from build123d import *

# Parameters (mm, degrees)
SKETCH1_W          = 51.5
SKETCH1_H          = 48.5
BASE_DEPTH         = 1.5
SKETCH1_6_W        = 51.5
SKETCH1_6_H        = 48.5
WALLS_DEPTH        = 17
SCREWS_START       = 11
SKETCH1_7_R        = 1
SKETCH1_7_W        = 1.5
SKETCH1_7_H        = 3
SKETCH1_7_H_2      = 4
SCREWS_DEPTH       = 1.5
TOP_START          = 15.5
SKETCH1_8_W        = 39.5
SKETCH1_8_H        = 3
SKETCH1_8_H_2      = 4
TOP_DEPTH          = 1.5
FILLET1_R          = 5
FILLET3_R          = 4
SKETCH2_R          = 4
CUT_EXTRUDE1_DEPTH = 1.5


with BuildPart() as part:
    # Sketch1 → base (new body)
    with BuildSketch(Plane(origin=(0, 0, 0), x_dir=(1, 0, 0), z_dir=(0, 1, 0))):
        with Locations((24.25, 22.75)):
            Rectangle(SKETCH1_W, SKETCH1_H)
    extrude(amount=BASE_DEPTH)

    # Sketch1<6> → walls (add)
    with BuildSketch(Plane(origin=(0, 0, 0), x_dir=(1, 0, 0), z_dir=(0, 1, 0))):
        with Locations((24.25, 22.75)):
            Rectangle(SKETCH1_6_W, SKETCH1_6_H)
        Polygon((4.5, 0), (0, 0), (0, 4.5), (0, 6), (0, 39.5), (0, 41), (0, 45.5), (4.5, 45.5), (6, 45.5), (42.5, 45.5), (44, 45.5), (48.5, 45.5), (48.5, 41), (48.5, 39.5), (48.5, 6), (48.5, 4.5), (48.5, 0), (44, 0), (42.5, 0), (6, 0), align=None, mode=Mode.SUBTRACT)
    extrude(amount=WALLS_DEPTH)

    # Sketch1<7> → screws (add)
    # profile 1 of 12: a face of its own
    with BuildSketch(Plane(origin=(0, 0, 0), x_dir=(1, 0, 0), z_dir=(0, 1, 0)).offset(SCREWS_START)):
        Polygon((44, 3), (44, 0), (48.5, 0), (48.5, 4.5), (44, 4.5), align=None)
        with Locations(Location((46.25, 2.25, 0), (0, 0, 270))):
            Circle(SKETCH1_7_R, mode=Mode.SUBTRACT)
    # profile 2 of 12: a face of its own
    with BuildSketch(Plane(origin=(0, 0, 0), x_dir=(1, 0, 0), z_dir=(0, 1, 0)).offset(SCREWS_START)):
        Polygon((42.5, 6), (42.5, 3), (44, 3), (44, 4.5), (48.5, 4.5), (48.5, 6), align=None)
    # profile 3 of 12: a face of its own
    with BuildSketch(Plane(origin=(0, 0, 0), x_dir=(1, 0, 0), z_dir=(0, 1, 0)).offset(SCREWS_START)):
        with Locations((43.25, 1.5)):
            Rectangle(SKETCH1_7_W, SKETCH1_7_H)
    # profile 4 of 12: a face of its own
    with BuildSketch(Plane(origin=(0, 0, 0), x_dir=(1, 0, 0), z_dir=(0, 1, 0)).offset(SCREWS_START)):
        Polygon((44, 41.5), (42.5, 41.5), (42.5, 39.5), (48.5, 39.5), (48.5, 41), (44, 41), align=None)
    # profile 5 of 12: a face of its own
    with BuildSketch(Plane(origin=(0, 0, 0), x_dir=(1, 0, 0), z_dir=(0, 1, 0)).offset(SCREWS_START)):
        Polygon((44, 45.5), (44, 41.5), (44, 41), (48.5, 41), (48.5, 45.5), align=None)
        with Locations(Location((46.25, 43.25, 0), (0, 0, 270))):
            Circle(SKETCH1_7_R, mode=Mode.SUBTRACT)
    # profile 6 of 12: a face of its own
    with BuildSketch(Plane(origin=(0, 0, 0), x_dir=(1, 0, 0), z_dir=(0, 1, 0)).offset(SCREWS_START)):
        with Locations((43.25, 43.5)):
            Rectangle(SKETCH1_7_W, SKETCH1_7_H_2)
    # profile 7 of 12: a face of its own
    with BuildSketch(Plane(origin=(0, 0, 0), x_dir=(1, 0, 0), z_dir=(0, 1, 0)).offset(SCREWS_START)):
        Polygon((0, 41), (0, 39.5), (6, 39.5), (6, 41.5), (4.5, 41.5), (4.5, 41), align=None)
    # profile 8 of 12: a face of its own
    with BuildSketch(Plane(origin=(0, 0, 0), x_dir=(1, 0, 0), z_dir=(0, 1, 0)).offset(SCREWS_START)):
        Polygon((0, 45.5), (0, 41), (4.5, 41), (4.5, 41.5), (4.5, 45.5), align=None)
        with Locations(Location((2.25, 43.25, 0), (0, 0, 270))):
            Circle(SKETCH1_7_R, mode=Mode.SUBTRACT)
    # profile 9 of 12: a face of its own
    with BuildSketch(Plane(origin=(0, 0, 0), x_dir=(1, 0, 0), z_dir=(0, 1, 0)).offset(SCREWS_START)):
        with Locations((5.25, 43.5)):
            Rectangle(SKETCH1_7_W, SKETCH1_7_H_2)
    # profile 10 of 12: a face of its own
    with BuildSketch(Plane(origin=(0, 0, 0), x_dir=(1, 0, 0), z_dir=(0, 1, 0)).offset(SCREWS_START)):
        Polygon((0, 4.5), (0, 0), (4.5, 0), (4.5, 3), (4.5, 4.5), align=None)
        with Locations(Location((2.25, 2.25, 0), (0, 0, 270))):
            Circle(SKETCH1_7_R, mode=Mode.SUBTRACT)
    # profile 11 of 12: a face of its own
    with BuildSketch(Plane(origin=(0, 0, 0), x_dir=(1, 0, 0), z_dir=(0, 1, 0)).offset(SCREWS_START)):
        Polygon((0, 6), (0, 4.5), (4.5, 4.5), (4.5, 3), (6, 3), (6, 6), align=None)
    # profile 12 of 12: a face of its own
    with BuildSketch(Plane(origin=(0, 0, 0), x_dir=(1, 0, 0), z_dir=(0, 1, 0)).offset(SCREWS_START)):
        with Locations((5.25, 1.5)):
            Rectangle(SKETCH1_7_W, SKETCH1_7_H)
    extrude(amount=SCREWS_DEPTH)

    # Sketch1<8> → top (add)
    with BuildSketch(Plane(origin=(0, 0, 0), x_dir=(1, 0, 0), z_dir=(0, 1, 0)).offset(TOP_START)):
        with Locations((24.25, 1.5)):
            Rectangle(SKETCH1_8_W, SKETCH1_8_H)
        with Locations((24.25, 43.5)):
            Rectangle(SKETCH1_8_W, SKETCH1_8_H_2)
    extrude(amount=TOP_DEPTH)

    # Fillet1
    # the kernel refuses this fillet: 5 mm, written as the material it adds along each edge
    with BuildSketch(Plane(origin=(0, 11, 0), x_dir=(0, -1, 0), z_dir=(1, 0, 0))) as fillet1_piece_1_section:
        with BuildLine():
            CenterArc((FILLET1_R, FILLET1_R), FILLET1_R, 180, 90)
            Line((0, FILLET1_R), (0, 0))
            Line((0, 0), (FILLET1_R, 0))
        make_face()
    fillet1_piece_1 = extrude(amount=6, mode=Mode.PRIVATE)
    fillet1_piece_1 = fillet1_piece_1 - Plane(origin=(2.25, 9.80856061, -2.25), x_dir=(0, 0, 1), z_dir=(0, -1, 0)) * Cylinder(1, 33, mode=Mode.PRIVATE)
    add(fillet1_piece_1)
    with BuildSketch(Plane(origin=(0, 11, -6), x_dir=(0, -1, 0), z_dir=(0, 0, 1))) as fillet1_piece_2_section:
        with BuildLine():
            CenterArc((FILLET1_R, FILLET1_R), FILLET1_R, 180, 90)
            Line((0, FILLET1_R), (0, 0))
            Line((0, 0), (FILLET1_R, 0))
        make_face()
    fillet1_piece_2 = extrude(amount=6, mode=Mode.PRIVATE)
    fillet1_piece_2 = fillet1_piece_2 - Plane(origin=(2.25, 9.808553236, -2.25), x_dir=(0, 0, 1), z_dir=(0, -1, 0)) * Cylinder(1, 32, mode=Mode.PRIVATE)
    add(fillet1_piece_2)
    with BuildSketch(Plane(origin=(0, 11, -45.5), x_dir=(0, -1, 0), z_dir=(0, 0, 1))) as fillet1_piece_3_section:
        with BuildLine():
            CenterArc((FILLET1_R, FILLET1_R), FILLET1_R, 180, 90)
            Line((0, FILLET1_R), (0, 0))
            Line((0, 0), (FILLET1_R, 0))
        make_face()
    fillet1_piece_3 = extrude(amount=6, mode=Mode.PRIVATE)
    fillet1_piece_3 = fillet1_piece_3 - Plane(origin=(2.25, 9.808553112, -43.25), x_dir=(0, 0, 1), z_dir=(0, -1, 0)) * Cylinder(1, 32, mode=Mode.PRIVATE)
    add(fillet1_piece_3)
    with BuildSketch(Plane(origin=(0, 11, -45.5), x_dir=(0, -1, 0), z_dir=(1, 0, 0))) as fillet1_piece_4_section:
        with BuildLine():
            CenterArc((FILLET1_R, -FILLET1_R), FILLET1_R, 90, 90)
            Line((0, -FILLET1_R), (0, 0))
            Line((0, 0), (FILLET1_R, 0))
        make_face()
    fillet1_piece_4 = extrude(amount=6, mode=Mode.PRIVATE)
    fillet1_piece_4 = fillet1_piece_4 - Plane(origin=(2.25, 9.808558943, -43.25), x_dir=(0, 0, 1), z_dir=(0, -1, 0)) * Cylinder(1, 33, mode=Mode.PRIVATE)
    add(fillet1_piece_4)
    with BuildSketch(Plane(origin=(48.5, 11, -45.5), x_dir=(0, -1, 0), z_dir=(-1, 0, 0))) as fillet1_piece_5_section:
        with BuildLine():
            CenterArc((FILLET1_R, FILLET1_R), FILLET1_R, 180, 90)
            Line((0, FILLET1_R), (0, 0))
            Line((0, 0), (FILLET1_R, 0))
        make_face()
    fillet1_piece_5 = extrude(amount=6, mode=Mode.PRIVATE)
    fillet1_piece_5 = fillet1_piece_5 - Plane(origin=(46.25, 9.808558971, -43.25), x_dir=(0, 0, 1), z_dir=(0, -1, 0)) * Cylinder(1, 33, mode=Mode.PRIVATE)
    add(fillet1_piece_5)
    with BuildSketch(Plane(origin=(48.5, 11, -45.5), x_dir=(0, -1, 0), z_dir=(0, 0, 1))) as fillet1_piece_6_section:
        with BuildLine():
            CenterArc((FILLET1_R, -FILLET1_R), FILLET1_R, 90, 90)
            Line((0, -FILLET1_R), (0, 0))
            Line((0, 0), (FILLET1_R, 0))
        make_face()
    fillet1_piece_6 = extrude(amount=6, mode=Mode.PRIVATE)
    fillet1_piece_6 = fillet1_piece_6 - Plane(origin=(46.25, 9.808552814, -43.25), x_dir=(0, 0, 1), z_dir=(0, -1, 0)) * Cylinder(1, 33, mode=Mode.PRIVATE)
    add(fillet1_piece_6)
    with BuildSketch(Plane(origin=(48.5, 11, -6), x_dir=(0, -1, 0), z_dir=(0, 0, 1))) as fillet1_piece_7_section:
        with BuildLine():
            CenterArc((FILLET1_R, -FILLET1_R), FILLET1_R, 90, 90)
            Line((0, -FILLET1_R), (0, 0))
            Line((0, 0), (FILLET1_R, 0))
        make_face()
    fillet1_piece_7 = extrude(amount=6, mode=Mode.PRIVATE)
    fillet1_piece_7 = fillet1_piece_7 - Plane(origin=(46.25, 9.808552873, -2.25), x_dir=(0, 0, 1), z_dir=(0, -1, 0)) * Cylinder(1, 33, mode=Mode.PRIVATE)
    add(fillet1_piece_7)
    with BuildSketch(Plane(origin=(48.5, 11, 0), x_dir=(0, -1, 0), z_dir=(-1, 0, 0))) as fillet1_piece_8_section:
        with BuildLine():
            CenterArc((FILLET1_R, -FILLET1_R), FILLET1_R, 90, 90)
            Line((0, -FILLET1_R), (0, 0))
            Line((0, 0), (FILLET1_R, 0))
        make_face()
    fillet1_piece_8 = extrude(amount=6, mode=Mode.PRIVATE)
    fillet1_piece_8 = fillet1_piece_8 - Plane(origin=(46.25, 9.808560411, -2.25), x_dir=(0, 0, 1), z_dir=(0, -1, 0)) * Cylinder(1, 32, mode=Mode.PRIVATE)
    add(fillet1_piece_8)

    # Fillet3
    # the kernel refuses this fillet: 4 mm, written as the material it adds along each edge
    with BuildSketch(Plane(origin=(4.5, 15.5, 0), x_dir=(0, -1, 0), z_dir=(1, 0, 0))) as fillet3_piece_1:
        with BuildLine():
            CenterArc((3.872983346, 4), FILLET3_R, 194.477512186, 75.522487814)
            Line((0, 3), (0, 0))
            Line((0, 0), (3.872983346, 0))
        make_face()
    extrude(amount=39.5)
    with BuildSketch(Plane(origin=(44, 15.5, -45.5), x_dir=(0, -1, 0), z_dir=(-1, 0, 0))) as fillet3_piece_2:
        with BuildLine():
            CenterArc((FILLET3_R, FILLET3_R), FILLET3_R, 180, 90)
            Line((0, FILLET3_R), (0, 0))
            Line((0, 0), (FILLET3_R, 0))
        make_face()
    extrude(amount=39.5)

    # Sketch2 → Cut-Extrude1 (cut)
    with BuildSketch(Plane.XY.offset(1.5)):
        with Locations((24.25, 8.5)):
            Circle(SKETCH2_R)
    extrude(amount=-CUT_EXTRUDE1_DEPTH, mode=Mode.SUBTRACT)


solid = part.part
Can you work these out from the model? Positions are in its coordinate system, mm. A direction names the side the tool comes from. Round coordinates to 2 decimals unless told otherwise and drop trailing zeros. Write each loop counter-clockwise with the first axis right and the second up, starting at its lowest first coordinate (ties: lowest second). Pieces come first, ordered by that corner, then holes. Notation, with made-up numbers: M 60,33.5 L 68,33.5 A19 cw 68,64.5 Z; hole C 21.5,76.25 d9. An arc over 180 degrees is marked long. Use a Markdown table: item, result.
Item 1: I want a section at B-B (y = 3.25). List the corners of the cut face in (x, z) for me, and give its area (3 significant figures).
Found:
| item | result |
|---|---|
| outline | M -1.5,-47 L 50,-47 L 50,1.5 L -1.5,1.5 Z; hole M 0,-45.5 L 48.5,-45.5 L 48.5,0 L 0,0 Z |
| area | 291 mm2 |
Item 2: I want a section at D-D (x = 29.5). List the corners of the cut face in (y, z) for me, and give its area (3 significant figures).
Found:
| item | result |
|---|---|
| outline | M 0,-47 L 17,-47 L 17,-41.5 L 15.5,-41.5 A4 cw 11.5,-45.5 L 1.5,-45.5 L 1.5,0 L 11.63,0 A4 cw 15.5,-3 L 17,-3 L 17,1.5 L 0,1.5 Z |
| area | 136 mm2 |
Item 3: Which directions (+Z, -Z, +X, -X, +Y, -Y) give clear straight access to the entire face, cutting with the end or side of a thin tool? Please do faces 1 (the face through (44, 16, -44)), 2 (the face through (21.076, 6.066, 0.76)), 3 (the face through (6, 11, -3)).
Found:
| item | result |
|---|---|
| face 1 | +Y |
| face 2 | +Z |
| face 3 | none |
Item 4: For pin 1 Ø6 at (x, z) = (7, -10) entering from +Y; pin 2 Ø1.8 at (x, z) = (3, -41) entering from +Y; pin 3 Ø0.7 at (x, y) = (25, 12) entering from +Z, each with a flat end and sliding along its axis, tell me the tip position at first contact or that it passes through.
Found:
| item | result |
|---|---|
| pin 1 | stops at y = 1.5 |
| pin 2 | stops at y = 12.5 |
| pin 3 | stops at z = 0 |
Item 5: We'd pull the mould along X, two halves only. Please class faces 4 (the face through (2, 15, -45.5)), 5 (the face through (48.5, 9, -23)), 6 (the face through (24, 17, -43)), 7 (the face through (-1.5, 8, -22)): released by +X, released by -X, zero draft, split by the parting line, or undercut.
Found:
| item | result |
|---|---|
| face 4 | undercut |
| face 5 | undercut |
| face 6 | zero draft |
| face 7 | released by -X |
Item 6: I want a section at A-A (x = 24.25). List the corners of the cut face in (y, z) for me.
Found:
| item | result |
|---|---|
| outline | M 0,-47 L 17,-47 L 17,-41.5 L 15.5,-41.5 A4 cw 11.5,-45.5 L 1.5,-45.5 L 1.5,0 L 4.5,0 L 4.5,1.5 L 0,1.5 Z; M 11.63,0 A4 cw 15.5,-3 L 17,-3 L 17,1.5 L 12.5,1.5 L 12.5,0 Z |
Item 7: I want a section at C-C (z = -15). List the corners of the cut face in (x, y) for me.
Found:
| item | result |
|---|---|
| outline | M -1.5,0 L 50,0 L 50,17 L 48.5,17 L 48.5,1.5 L 0,1.5 L 0,17 L -1.5,17 Z |
Item 8: If I drill on line 1 along Z through (x, y) = (46.25, 10.35); line 2 along X through (y, z) = (11.5, -43.25); line 3 along Z through (x, y) = (30, 8), over which ranges is the centre line in solid material (lowest first)? Write a range as [from, to].
Found:
| item | result |
|---|---|
| line 1 | z = [-47, -44.25], [-42.25, -39.5], [-6, -3.25], [-1.25, 1.5] |
| line 2 | x = [-1.5, 1.25], [3.25, 6], [42.5, 45.25], [47.25, 50] |
| line 3 | z = [-47, -45.5], [0, 1.5] |
